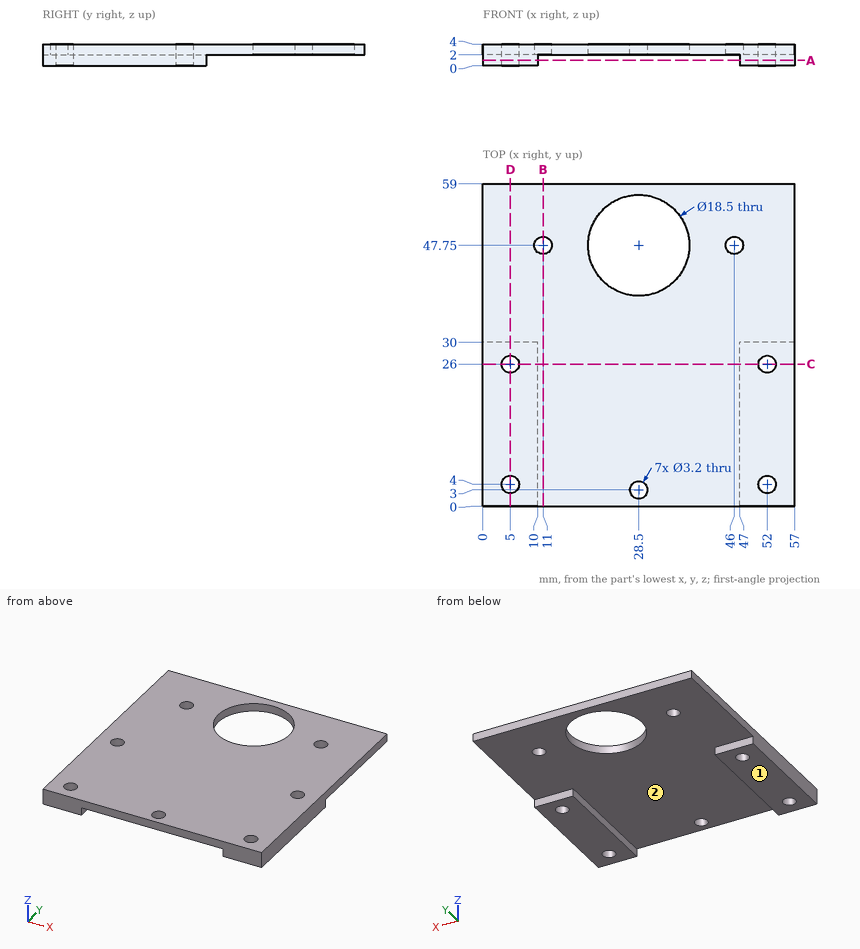
Design review of the part shown in the three views and the two pictorial views. Dimensions are in mm from the part's minimum x, y and z. Round coordinates to 2 decimals unless told otherwise and drop trailing zeros. Write each loop counter-clockwise with the first axis right and the second up, starting at its lowest first coordinate (ties: lowest second). Pieces come first, ordered by that corner, then holes. Notation, with made-up numbers: (5.5, -24.5) -> (14.5, -24.5) arc R8 cw to (14.5, -19.5) -> close; hole circle Ø9 at (34.25, -28). An arc over 180 degrees is marked (long way). One line per question, with ' | ' between items. Start each with the question number.
1) Add section D-D (x = 5). Write out the cut boundary in (y, z), and give its area (3 significant figures).
2) Add section B-B (x = 11). Write out the cut boundary in (y, z).
3) Add section A-A (z = 1). Write out the cut boundary in (x, y).
4) Mouldability with a two-part tool opening along X and no side actions: class the marked faces 1 and 2 as +X half, -X half, draft (parallel to the pull), parting line (faces both ways), or undercut.
5) Add section C-C (y = 26). Write out the cut boundary in (x, z), and give its area (3 significant figures).
6) Wall thickness on line 1 along Y through (x, z) = (5, 3.1); line 2 along Y through (x, z) = (51, 2.35); line 3 along Y through (x, z) = (11, 2.9): over which ranges is each line inside the solid? List them lowest first.
7) For pin 1 Ø4 at (x, y) = (28.5, 3) entering from -Z; pin 2 Ø1.6 at (x, z) = (6.5, 0.5) entering from +Y, all flat-tipped, find the tip position at first contact; note any pin that passes through.
Reported:
1) outline: (0, 0) -> (2.4, 0) -> (2.4, 4) -> (0, 4) -> close; (5.6, 0) -> (24.4, 0) -> (24.4, 4) -> (5.6, 4) -> close; (27.6, 0) -> (30, 0) -> (30, 2) -> (59, 2) -> (59, 4) -> (27.6, 4) -> close | area: 152 mm²
2) outline: (0, 2) -> (46.15, 2) -> (46.15, 4) -> (0, 4) -> close; (49.35, 2) -> (59, 2) -> (59, 4) -> (49.35, 4) -> close
3) outline: (0, 0) -> (10, 0) -> (10, 30) -> (0, 30) -> close; (47, 0) -> (57, 0) -> (57, 30) -> (47, 30) -> close; hole circle Ø3.2 at (5, 4); hole circle Ø3.2 at (5, 26); hole circle Ø3.2 at (52, 4); hole circle Ø3.2 at (52, 26)
4) face 1: draft | face 2: undercut
5) outline: (0, 0) -> (3.4, 0) -> (3.4, 4) -> (0, 4) -> close; (6.6, 0) -> (10, 0) -> (10, 2) -> (47, 2) -> (47, 0) -> (50.4, 0) -> (50.4, 4) -> (6.6, 4) -> close; (53.6, 0) -> (57, 0) -> (57, 4) -> (53.6, 4) -> close | area: 128 mm²
6) line 1: y = 0 to 2.4, 5.6 to 24.4, 27.6 to 59 | line 2: y = 0 to 2.75, 5.25 to 24.75, 27.25 to 59 | line 3: y = 0 to 46.15, 49.35 to 59
7) pin 1: stops at z = 2 | pin 2: stops at y = 30
